Read the model definition and answer for the solid it produces. Units are mm, in the model's axes. Give positions to 0.01 mm unless a question says otherwise; leave off trailing zeros. Write each loop counter-clockwise with the first axis right and the second up, starting at its lowest first coordinate (ties: lowest second). Pieces come first, ordered by that corner, then holes. Notation, with made-up numbers: (13.5, -19) - (24.5, -19) arc R4 cw to (24.5, -12) - close; hole circle Ø8 at (46, 65.25). An arc over 180 degrees is marked (long way). Answer as CSV lines item,"result".
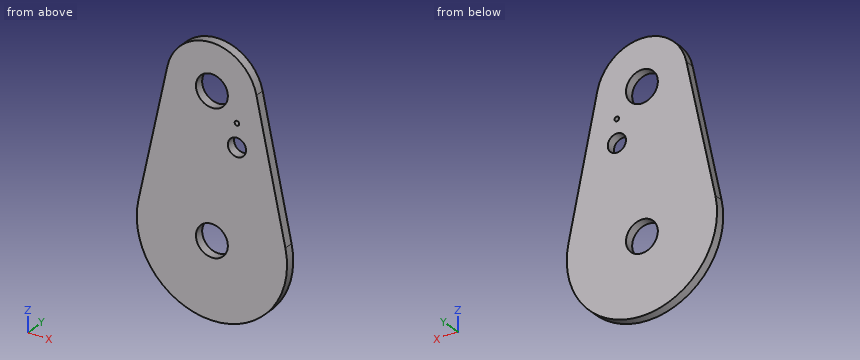
```python
from build123d import *

# Parameters (mm, degrees)
SKETCH_R   = 7
SKETCH_R_2 = 4
SKETCH_R_3 = 1
PAD_DEPTH  = 4


with BuildPart() as part:
    # Sketch → Pad (new body)
    with BuildSketch(Plane.XZ):
        with BuildLine():
            Line((-19.555423, 66.193498), (-32.26643, 6.919355))
            ThreePointArc((-32.26643, 6.919355), (0, -33), (32.26643, 6.919355))
            Line((19.555402, 66.193599), (32.26643, 6.919355))
            ThreePointArc((19.555402, 66.193599), (-5.1e-05, 82), (-19.555423, 66.193498))
        make_face()
        with Locations((0, 62)):
            Circle(SKETCH_R, mode=Mode.SUBTRACT)
        Circle(SKETCH_R, mode=Mode.SUBTRACT)
        with Locations((11, 42)):
            Circle(SKETCH_R_2, mode=Mode.SUBTRACT)
        with Locations((11, 52)):
            Circle(SKETCH_R_3, mode=Mode.SUBTRACT)
    extrude(amount=PAD_DEPTH)


solid = part.part
```
(1) Find the intervals of material crossed by L1, parallel to Z at x = 0, y = -2.85; L2, parallel to Z at x = 11, y = -1.45; L3, parallel to X at y = -0.4, z = 3, in increasing order.
Worked out:
L1,"z = -33 to -7, 7 to 55, 69 to 82"
L2,"z = -31.11 to 38, 46 to 51, 53 to 78.7"
L3,"x = -32.86 to -6.32, 6.32 to 32.86"
(2) A cutting plane is placed at C-C (y = -1). Write down the section's boundary in (x, z).
Worked out:
outline,"(-32.27, 6.92) arc R33 ccw (long way) to (32.27, 6.92) - (19.56, 66.19) arc R20 ccw to (-19.56, 66.19) - close; hole circle Ø14 at (0, 0); hole circle Ø14 at (0, 62); hole circle Ø8 at (11, 42); hole circle Ø2 at (11, 52)"
(3) A cutting plane is placed at B-B (x = 0). Write down the section's boundary in (y, z), and give its area (3 significant figures).
Worked out:
outline,"(-4, -33) - (0, -33) - (0, -7) - (-4, -7) - close; (-4, 7) - (0, 7) - (0, 55) - (-4, 55) - close; (-4, 69) - (0, 69) - (0, 82) - (-4, 82) - close"
area,"348 mm^2"
(4) Each of these flat-tipped pins is pushed along its axis until it touches: P1, Ø1.5, axis at y = -0.5, z = 65, coming from the -X side; P2, Ø7, axis at x = 11, z = 42, coming from the +Y side. Where does it stop, or does it pass through?
Worked out:
P1,"stops at x = -19.97"
P2,"passes through"
(5) A cutting plane is placed at A-A (z = 0). Write down the section's boundary in (x, y).
Worked out:
outline,"(-33, -4) - (-7, -4) - (-7, 0) - (-33, 0) - close; (7, -4) - (33, -4) - (33, 0) - (7, 0) - close"
(6) A cutting plane is placed at D-D (z = 42). Write down the section's boundary in (x, y), and give its area (3 significant figures).
Worked out:
outline,"(-24.74, -4) - (7, -4) - (7, 0) - (-24.74, 0) - close; (15, -4) - (24.74, -4) - (24.74, 0) - (15, 0) - close"
area,"166 mm^2"
